Geometry check sheet. Reference: drawing and pictorial views, mm from the part's lowest x, y, z. Give positions to 0.01 mm unless a question says otherwise; leave off trailing zeros. Write each loop counter-clockwise with the first axis right and the second up, starting at its lowest first coordinate (ties: lowest second). Pieces come first, ordered by that corner, then holes. Notation, with made-up numbers: (50, 18.25) -> (87, 18.25) arc R20 ccw to (87, 42.25) -> close; hole circle Ø8 at (7.25, -26). An arc over 180 degrees is marked (long way). Return JSON: item names as keys, results as strings.
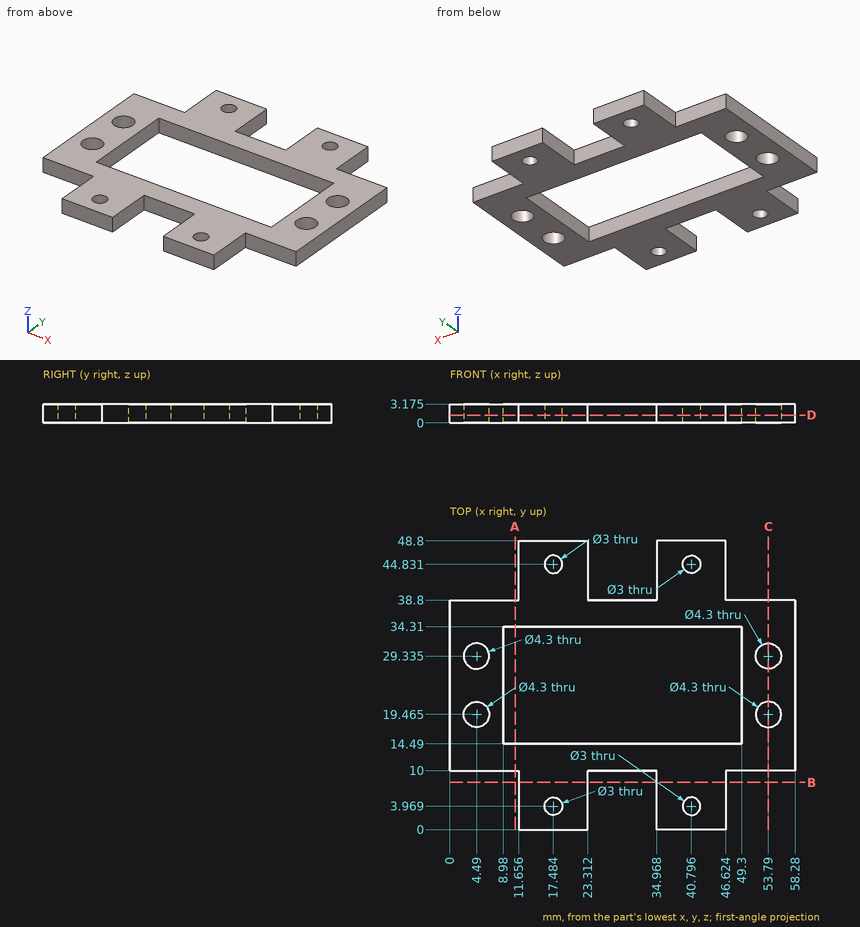
(1) Depth check by flat-ended pin: pin 1 Ø1.8 at (x, y) = (40.8, 44.83) entering from +Z; pin 2 Ø1.6 at (y, z) = (5, 1) entering from +X; pin 3 Ø1 at (x, z) = (53.5, 1.5) entering from -Y; pin 4 Ø1 at (y, z) = (4.5, 1) entering from -X. Enter the tip coordinate at first touch or a pass-through.
Reply:
{"pin 1": "through", "pin 2": "x = 46.62", "pin 3": "y = 10", "pin 4": "x = 11.66"}
(2) Cross-section at C-C on x = 53.79. Enter the section's corners in (y, z) (1 decimal).
Reply:
{"outline": "(10, 0) -> (17.3, 0) -> (17.3, 3.2) -> (10, 3.2) -> close; (21.6, 0) -> (27.2, 0) -> (27.2, 3.2) -> (21.6, 3.2) -> close; (31.5, 0) -> (38.8, 0) -> (38.8, 3.2) -> (31.5, 3.2) -> close"}
(3) Cross-section at B-B on y = 8. Enter the section's corners in (x, z) (1 decimal), then the cut area to 3 significant figures.
Reply:
{"outline": "(11.7, 0) -> (23.3, 0) -> (23.3, 3.2) -> (11.7, 3.2) -> close; (35, 0) -> (46.6, 0) -> (46.6, 3.2) -> (35, 3.2) -> close", "area": "74.0 mm^2"}
(4) Cross-section at A-A on x = 11. Enter the section's corners in (y, z) (1 decimal).
Reply:
{"outline": "(10, 0) -> (14.5, 0) -> (14.5, 3.2) -> (10, 3.2) -> close; (34.3, 0) -> (38.8, 0) -> (38.8, 3.2) -> (34.3, 3.2) -> close"}
(5) Thickness scan on L1, parallel to Y at x = 53.79, z = 0.7 (1 decimal); L2, parallel to Y at x = 16.5, z = 1.7; L3, parallel to X at y = 4, z = 2.1. Record the ranges inside material, lowest first.
Reply:
{"L1": "10 to 17.3, 21.6 to 27.2, 31.5 to 38.8", "L2": "0 to 2.84, 5.1 to 14.49, 34.31 to 43.7, 45.96 to 48.8", "L3": "11.66 to 15.98, 18.98 to 23.31, 34.97 to 39.3, 42.3 to 46.62"}
(6) Cross-section at D-D on z = 1.3. State how many separate pieces and enclosed holes the cut face has, then the cut area to 3 significant figures.
Reply:
{"separate pieces": "1", "enclosed holes": "9", "area": "1,260 mm^2"}
